The listing builds one solid part. Answer for the finished solid, in the listing's coordinates (mm). Face numbers are marked on the shaded views. A direction names the side the tool comes from. Give positions to 0.01 mm unless a question says otherwise; leave off trailing zeros. Order: outer loops, then holes, each group sorted by start corner. A loop starts at its lowest first (then second) coordinate and runs counter-clockwise, first axis right, second up. Notation, with made-up numbers: (58.5, 40) -> (62.5, 40) arc R18 ccw to (62.5, 61) -> close; hole circle Ø6 at (31.5, 66.5). An arc over 180 degrees is marked (long way). Answer as a JSON object with one key per item and string values. Group by question number.
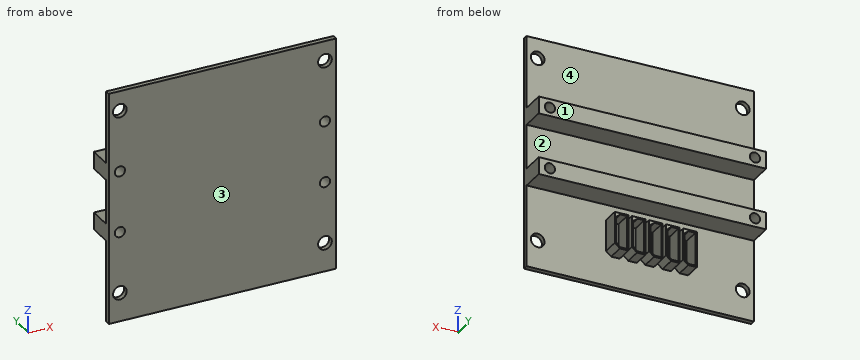
```python
from build123d import *

# Parameters (mm, degrees)
SKETCH1_W               = 66.5
SKETCH1_H               = 68.25
BOSS_EXTRUDE1_DEPTH     = 1.5
CUT_EXTRUDE1_DEPTH      = 48.668942982
CUT_EXTRUDE1_DEPTH_BACK = 48.668942982
SKETCH3_R               = 2
SKETCH3_R_2             = 1.5
BOSS_EXTRUDE2_DEPTH     = 5
SKETCH6_W               = 66.5
SKETCH6_H               = 5
BOSS_EXTRUDE3_DEPTH     = 7
CUT_EXTRUDE2_DEPTH      = 49.397604538
CUT_EXTRUDE2_DEPTH_BACK = 49.397604538
SKETCH7_R               = 1.5


with BuildPart() as part:
    # Sketch1 → Boss-Extrude1 (new body)
    with BuildSketch(Plane(origin=(0, 0, 0), x_dir=(1, 0, 0), z_dir=(0, 1, 0))):
        Rectangle(SKETCH1_W, SKETCH1_H)
    extrude(amount=BOSS_EXTRUDE1_DEPTH)

    # Sketch3 → Cut-Extrude1 (cut, two sides: drawn at the far end of the back side and taken through both)
    with BuildSketch(Plane(origin=(0, 1.5, 0), x_dir=(1, 0, 0), z_dir=(0, 1, 0)).offset(-CUT_EXTRUDE1_DEPTH_BACK)):
        with Locations(Location((-30, -28.317585536, 0), (0, 0, 270))):
            Circle(SKETCH3_R)
        with Locations(Location((30, -28.317585536, 0), (0, 0, 270))):
            Circle(SKETCH3_R)
        with Locations(Location((30, 25.682414464, 0), (0, 0, 270))):
            Circle(SKETCH3_R)
        with Locations(Location((-30, 25.682414464, 0), (0, 0, 270))):
            Circle(SKETCH3_R)
        with Locations(Location((30, 7.682414464, 0), (0, 0, 270))):
            Circle(SKETCH3_R_2)
        with Locations(Location((30, -10.317585536, 0), (0, 0, 270))):
            Circle(SKETCH3_R_2)
        with Locations(Location((-30, -10.317585536, 0), (0, 0, 270))):
            Circle(SKETCH3_R_2)
        with Locations(Location((-30, 7.682414464, 0), (0, 0, 270))):
            Circle(SKETCH3_R_2)
    extrude(amount=CUT_EXTRUDE1_DEPTH + CUT_EXTRUDE1_DEPTH_BACK, mode=Mode.SUBTRACT)

    # Sketch5 → Boss-Extrude2 (add)
    # profile 1 of 5: a face of its own
    with BuildSketch(Plane(origin=(0, 1.5, 0), x_dir=(1, 0, 0), z_dir=(0, 1, 0))):
        Polygon((-14.006270714, 25.182414464), (-11.506270714, 25.182414464), (-10.006270714, 23.882414464), (-10.006270714, 14.682414464), (-14.006270714, 14.682414464), align=None)
        Polygon((-10.406270714, 23.699762911), (-10.406270714, 15.999762911), (-11.656270714, 15.082414464), (-13.606270714, 15.082414464), (-13.606270714, 24.782414464), (-11.655484044, 24.782414464), align=None, mode=Mode.SUBTRACT)
    # profile 2 of 5: a face of its own
    with BuildSketch(Plane(origin=(0, 1.5, 0), x_dir=(1, 0, 0), z_dir=(0, 1, 0))):
        Polygon((-9.006270714, 25.182414464), (-6.506270714, 25.182414464), (-5.006270714, 23.882414464), (-5.006270714, 14.682414464), (-9.006270714, 14.682414464), align=None)
        Polygon((-5.406270714, 23.699762911), (-5.406270714, 15.999762911), (-6.656270714, 15.082414464), (-8.606270714, 15.082414464), (-8.606270714, 24.782414464), (-6.655484044, 24.782414464), align=None, mode=Mode.SUBTRACT)
    # profile 3 of 5: a face of its own
    with BuildSketch(Plane(origin=(0, 1.5, 0), x_dir=(1, 0, 0), z_dir=(0, 1, 0))):
        Polygon((-4.006270714, 25.182414464), (-1.506270714, 25.182414464), (-0.006270714, 23.882414464), (-0.006270714, 14.682414464), (-4.006270714, 14.682414464), align=None)
        Polygon((-0.406270714, 23.699762911), (-0.406270714, 15.999762911), (-1.656270714, 15.082414464), (-3.606270714, 15.082414464), (-3.606270714, 24.782414464), (-1.655484044, 24.782414464), align=None, mode=Mode.SUBTRACT)
    # profile 4 of 5: a face of its own
    with BuildSketch(Plane(origin=(0, 1.5, 0), x_dir=(1, 0, 0), z_dir=(0, 1, 0))):
        Polygon((0.993729286, 25.182414464), (3.493729286, 25.182414464), (4.993729286, 23.882414464), (4.993729286, 14.682414464), (0.993729286, 14.682414464), align=None)
        Polygon((4.593729286, 23.699762911), (4.593729286, 15.999762911), (3.343729286, 15.082414464), (1.393729286, 15.082414464), (1.393729286, 24.782414464), (3.344515956, 24.782414464), align=None, mode=Mode.SUBTRACT)
    # profile 5 of 5: a face of its own
    with BuildSketch(Plane(origin=(0, 1.5, 0), x_dir=(1, 0, 0), z_dir=(0, 1, 0))):
        Polygon((5.993729286, 25.182414464), (8.493729286, 25.182414464), (9.993729286, 23.882414464), (9.993729286, 14.682414464), (5.993729286, 14.682414464), align=None)
        Polygon((9.593729286, 23.699762911), (9.593729286, 15.999762911), (8.343729286, 15.082414464), (6.393729286, 15.082414464), (6.393729286, 24.782414464), (8.344515956, 24.782414464), align=None, mode=Mode.SUBTRACT)
    extrude(amount=BOSS_EXTRUDE2_DEPTH)

    # Sketch6 → Boss-Extrude3 (add)
    with BuildSketch(Plane(origin=(0, 1.5, 0), x_dir=(1, 0, 0), z_dir=(0, 1, 0))):
        with Locations((0, 7.682414464)):
            Rectangle(SKETCH6_W, SKETCH6_H)
        with Locations((0, -10.317585536)):
            Rectangle(SKETCH6_W, SKETCH6_H)
    extrude(amount=BOSS_EXTRUDE3_DEPTH)

    # Sketch7 → Cut-Extrude2 (cut, two sides: drawn at the far end of the back side and taken through both)
    with BuildSketch(Plane(origin=(0, 8.5, 0), x_dir=(1, 0, 0), z_dir=(0, 1, 0)).offset(-CUT_EXTRUDE2_DEPTH_BACK)):
        with Locations(Location((-30, 7.682414464, 0), (0, 0, 270))):
            Circle(SKETCH7_R)
        with Locations(Location((-30, -10.317585536, 0), (0, 0, 270))):
            Circle(SKETCH7_R)
        with Locations(Location((30, -10.317585536, 0), (0, 0, 270))):
            Circle(SKETCH7_R)
        with Locations(Location((30, 7.682414464, 0), (0, 0, 270))):
            Circle(SKETCH7_R)
    extrude(amount=CUT_EXTRUDE2_DEPTH + CUT_EXTRUDE2_DEPTH_BACK, mode=Mode.SUBTRACT)


solid = part.part
```
(1) A cutting plane is placed at C-C (x = 19). Determine the outline of the cut face in (y, z) (3 decimals).
(2) A cutting plane is placed at D-D (z = 21). Determine the outline of the cut face in (x, y), and give its area (4 significant figures).
(3) For a pull along Z with two mould halves and no side action, classify the marked faces 1 and 2 as +Z half, -Z half, draft (parallel to the pull), parting line (faces both ways), or undercut.
(4) A cutting plane is placed at A-A (x = 30). Determine the outline of the cut face in (y, z) (3 decimals), and give its area (3 significant figures).
(5) A cutting plane is placed at B-B (y = 5.5). State how many separate pieces and enclosed holes the cut face has, and give its area (3 significant figures).
(6) Find the intervals of material crossed by line 1 along Z through (x, y) = (-30, 4); line 2 along Z through (x, y) = (-30, 1) (3 decimals); line 3 along Z through (x, y) = (-27, 7), in increasing order. Write a range as [from, to].
(7) Flat-ended cylindrical pins translate along their axes: pin 1 Ø2 at (x, y) = (-12.5, 4.5) entering from +Z; pin 2 Ø1 at (x, z) = (3, -20.5) entering from +Y; pin 3 Ø1 at (x, y) = (17, 2.5) entering from -Z; pin 4 Ø1.8 at (x, z) = (-30, 10.32) entering from -Y. Find the tip coordinate at first contact, or state that the pin passes through.
(8) Which of the six approach directions +Z, -Z, +X, -X, +Y, -Y give full straight-line access (tool end or side, diameter ignored) to the marked faces 3 and 4?
Check sheet entries:
{
 "1": {"outline": "(0, -34.125) -> (1.5, -34.125) -> (1.5, -10.182) -> (8.5, -10.182) -> (8.5, -5.182) -> (1.5, -5.182) -> (1.5, 7.818) -> (8.5, 7.818) -> (8.5, 12.818) -> (1.5, 12.818) -> (1.5, 34.125) -> (0, 34.125) -> close"},
 "2": {"outline": "(-33.25, 0) -> (33.25, 0) -> (33.25, 1.5) -> (-33.25, 1.5) -> close", "area": "99.75 mm2"},
 "3": {"face 1": "draft", "face 2": "undercut"},
 "4": {"outline": "(0, -34.125) -> (1.5, -34.125) -> (1.5, -27.682) -> (0, -27.682) -> close; (0, -23.682) -> (1.5, -23.682) -> (1.5, -10.182) -> (8.5, -10.182) -> (8.5, -9.182) -> (0, -9.182) -> close; (0, -6.182) -> (8.5, -6.182) -> (8.5, -5.182) -> (1.5, -5.182) -> (1.5, 7.818) -> (8.5, 7.818) -> (8.5, 8.818) -> (0, 8.818) -> close; (0, 11.818) -> (8.5, 11.818) -> (8.5, 12.818) -> (1.5, 12.818) -> (1.5, 26.318) -> (0, 26.318) -> close; (0, 30.318) -> (1.5, 30.318) -> (1.5, 34.125) -> (0, 34.125) -> close", "area": "109 mm2"},
 "5": {"separate pieces": "7", "enclosed holes": "9", "area": "693 mm2"},
 "6": {"line 1": "z = [-10.18, -9.18], [-6.18, -5.18], [7.82, 8.82], [11.82, 12.82]", "line 2": "z = [-34.125, -27.682], [-23.682, -9.182], [-6.182, 8.818], [11.818, 26.318], [30.318, 34.125]", "line 3": "z = [-10.18, -5.18], [7.82, 12.82]"},
 "7": {"pin 1": "stops at z = 12.82", "pin 2": "stops at y = 1.5", "pin 3": "stops at z = -10.18", "pin 4": "passes through"},
 "8": {"face 3": "+Z, -Z, +X, -X, -Y", "face 4": "+Z, +X, -X, +Y"}
}
